```python
from build123d import *

# Parameters (mm, degrees)
SKETCH1_W           = 114.3
SKETCH1_H           = 225.425
BOSS_EXTRUDE1_DEPTH = 50.8
SKETCH2_W           = 107.95
SKETCH2_H           = 25.4
CUT_EXTRUDE1_DEPTH  = 38.1
SKETCH4_R           = 1.7145
CUT_EXTRUDE2_DEPTH  = 114.3


with BuildPart() as part:
    # Sketch1 → Boss-Extrude1 (new body)
    with BuildSketch(Plane.XY):
        with Locations((3.533467742, -71.539919355)):
            Rectangle(SKETCH1_W, SKETCH1_H)
    extrude(amount=BOSS_EXTRUDE1_DEPTH)

    # Sketch2 → Cut-Extrude1 (cut)
    with BuildSketch(Plane.XY.offset(50.8)):
        with Locations((3.533467742, -171.552419355)):
            Rectangle(SKETCH2_W, SKETCH2_H)
    extrude(amount=-CUT_EXTRUDE1_DEPTH, mode=Mode.SUBTRACT)

    # Sketch4 → Cut-Extrude2 (cut)
    with BuildSketch(Plane(origin=(60.683467742, 0, 0), x_dir=(0, 0, -1), z_dir=(1, 0, 0))):
        with Locations(Location((-12.7, -152.502419355, 0), (0, 0, 90))):
            Circle(SKETCH4_R)
        with Locations(Location((-38.1, -152.502419355, 0), (0, 0, 90))):
            Circle(SKETCH4_R)
        with Locations(Location((-38.1, -0.102419355, 0), (0, 0, 90))):
            Circle(SKETCH4_R)
        with Locations(Location((-12.7, -0.102419355, 0), (0, 0, 90))):
            Circle(SKETCH4_R)
    extrude(amount=-CUT_EXTRUDE2_DEPTH, mode=Mode.SUBTRACT)


solid = part.part
```
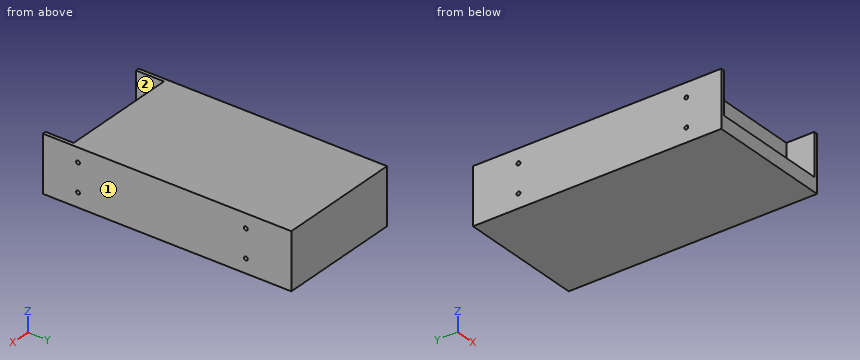
Part model, mm, in its own coordinate system. Face numbers are marked on the shaded views. A direction names the side the tool comes from. Coordinates: 2 decimals unless noted, no trailing zeros. Order: outer loops, then holes, each group sorted by start corner. A loop starts at its lowest first (then second) coordinate and runs counter-clockwise, first axis right, second up. Notation, with made-up numbers: (31.25, -18) -> (89.25, -18) arc R27 ccw to (89.25, 4) -> close; hole circle Ø5 at (-38, 15). An arc over 180 degrees is marked (long way). Put each result on its own line as item: value. Start each with the question number.
(1) Which spindle directions (+Z, -Z, +X, -X, +Y, -Y) get a long thin tool onto all of the face, cutting with end or side? Do the marked faces 1 and 2. Say none if no direction does.
(2) Pin check, flat tips, straight feed: pin 1 Ø2 at (y, z) = (-0.1, 12.7) entering from +X; pin 2 Ø4 at (x, z) = (30.5, 18) entering from -Y; pin 3 Ø7.5 at (x, y) = (10.5, -170.5) entering from +Z. Stop position of each tip, or through.
(3) Band-saw the part on B-B (y = -161). Give the cut face in (x, z), then the cut area to 3 significant figures.
(4) Probe line 1 along X through (y, z) = (-161.5, 20.5); line 2 along Z through (x, y) = (16, -175); line 3 along Y through (x, z) = (25.5, 16). List the from-to ranges inside material, lowest first. Write a range as [from, to].
(5) Band-saw the part on A-A (x = -25). Give the cut face in (y, z), then the cut area to 3 significant figures.
Determined:
1. face 1: +Z, -Z, +X, +Y, -Y
1. face 2: +Z, -Y
2. pin 1: passes through
2. pin 2: stops at y = -158.85
2. pin 3: stops at z = 12.7
3. outline: (-53.62, 0) -> (60.68, 0) -> (60.68, 50.8) -> (57.51, 50.8) -> (57.51, 12.7) -> (-50.44, 12.7) -> (-50.44, 50.8) -> (-53.62, 50.8) -> close
3. area: 1,690 mm²
4. line 1: x = [-53.62, -50.44], [57.51, 60.68]
4. line 2: z = [0, 12.7]
4. line 3: y = [-158.85, 41.17]
5. outline: (-184.25, 0) -> (41.17, 0) -> (41.17, 50.8) -> (-158.85, 50.8) -> (-158.85, 12.7) -> (-184.25, 12.7) -> close; hole circle Ø3.43 at (-152.5, 12.7); hole circle Ø3.43 at (-152.5, 38.1); hole circle Ø3.43 at (-0.1, 12.7); hole circle Ø3.43 at (-0.1, 38.1)
5. area: 10,400 mm²
